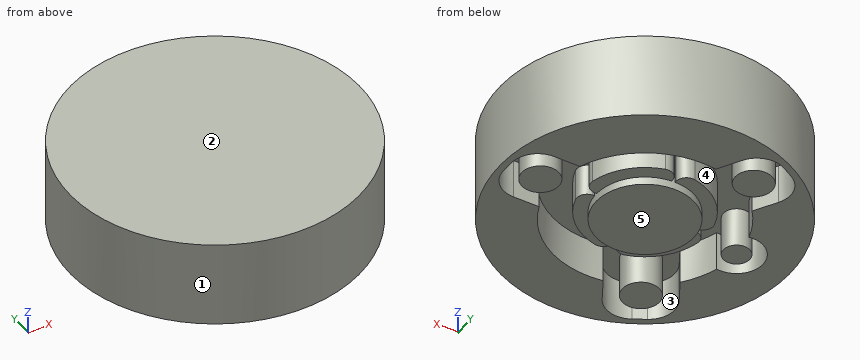
```python
from build123d import *

# Parameters (mm, degrees)
CYLINDER040_R     = 1
CYLINDER040_DEPTH = 10
CYLINDER037_R     = 3.7
CYLINDER037_DEPTH = 10
CYLINDER038_W     = 4.7
CYLINDER038_H     = 10
CYLINDER038_ANGLE = 86
FILLET003_R       = 0.79
ARRAY006_COUNT    = 4
CYLINDER036_R     = 1.4
CYLINDER036_DEPTH = 10
ARRAY004_COUNT    = 3
BOX003_W          = 10
BOX003_H          = 5
BOX003_DEPTH      = 3
FILLET002_R       = 2
ARRAY005_COUNT    = 3
CYLINDER035_R     = 7
CYLINDER035_DEPTH = 3
CYLINDER039_R     = 2
CYLINDER039_DEPTH = 3
CYLINDER042_R     = 11
CYLINDER042_DEPTH = 6.5


with BuildPart() as cylinder022:
    # Cylinder040 → Cylinder040 (new body)
    with BuildSketch(Plane(origin=(-7, 0, 0), x_dir=(1, 0, 0), z_dir=(0, 0, 1))):
        Circle(CYLINDER040_R)
    extrude(amount=CYLINDER040_DEPTH)


with BuildPart() as mountplateinnerhole002:
    # Cylinder037 → Cylinder037 (new body)
    with BuildSketch(Plane.XY):
        Circle(CYLINDER037_R)
    extrude(amount=CYLINDER037_DEPTH)


with BuildPart() as array006:
    # Cylinder038 → Cylinder038 (revolve)
    with BuildSketch(Plane(origin=(0, 0, 0.6), x_dir=(1, 0, 0), z_dir=(0, -1, 0))):
        with Locations((2.35, 5)):
            Rectangle(CYLINDER038_W, CYLINDER038_H)
    revolve(axis=Axis((0, 0, 0.6), (0, 0, 1)), revolution_arc=CYLINDER038_ANGLE)

    # Fillet003
    fillet003_edges = [array006.edges().sort_by_distance(p)[0] for p in [
        (0.327855, 4.688551, 5.6),
        (4.7, 0, 5.6),
    ]]
    fillet(fillet003_edges, radius=FILLET003_R)

    # Array006: Array006 ×4 about axis
    array006_axis = Axis((0, 0, 0), (0, 0, 1))


with BuildPart() as array006_1:
    add(array006.part)
    for i in range(1, ARRAY006_COUNT):
        add(array006.part.rotate(array006_axis, i * 360 / ARRAY006_COUNT))


with BuildPart() as fusion011:
    # Cylinder036 → Cylinder036 (new body)
    with BuildSketch(Plane(origin=(8, 0, 0), x_dir=(1, 0, 0), z_dir=(0, 0, 1))):
        Circle(CYLINDER036_R)
    extrude(amount=CYLINDER036_DEPTH)

    # Array004: Fusion011 ×3 about axis
    array004_axis = Axis((0, 0, 0), (0, 0, 1))


with BuildPart() as fusion011_1:
    add(fusion011.part)
    for i in range(1, ARRAY004_COUNT):
        add(fusion011.part.rotate(array004_axis, i * 360 / ARRAY004_COUNT))

    # Fusion011: union Cylinder022, MountPlateInnerHole002, Array006
    add(cylinder022.part)
    add(mountplateinnerhole002.part)
    add(array006_1.part)


with BuildPart() as array005:
    # Box003 → Box003 (new body)
    with BuildSketch(Plane(origin=(0.5, -2.5, 0), x_dir=(1, 0, 0), z_dir=(0, 0, 1))):
        with Locations((5, 2.5)):
            Rectangle(BOX003_W, BOX003_H)
    extrude(amount=BOX003_DEPTH)

    # Fillet002
    fillet002_edges = [array005.edges().sort_by_distance(p)[0] for p in [
        (10.5, -2.5, 1.5),
        (10.5, 2.5, 1.5),
    ]]
    fillet(fillet002_edges, radius=FILLET002_R)

    # Array005: Array005 ×3 about axis
    array005_axis = Axis((0, 0, 0), (0, 0, 1))


with BuildPart() as array005_1:
    add(array005.part)
    for i in range(1, ARRAY005_COUNT):
        add(array005.part.rotate(array005_axis, i * 360 / ARRAY005_COUNT))


with BuildPart() as mountplatebody002:
    # Cylinder035 → Cylinder035 (new body)
    with BuildSketch(Plane.XY):
        Circle(CYLINDER035_R)
    extrude(amount=CYLINDER035_DEPTH)


with BuildPart() as cut011:
    # Cylinder039 → Cylinder039 (new body)
    with BuildSketch(Plane(origin=(-7, 0, 0), x_dir=(1, 0, 0), z_dir=(0, 0, 1))):
        Circle(CYLINDER039_R)
    extrude(amount=CYLINDER039_DEPTH)

    # Fusion010: union Array005, MountPlateBody002
    add(array005_1.part)
    add(mountplatebody002.part)

    # Cut011: cut Fusion011
    add(fusion011_1.part, mode=Mode.SUBTRACT)


with BuildPart() as cut012:
    # Cylinder042 → Cylinder042 (new body)
    with BuildSketch(Plane.XY):
        Circle(CYLINDER042_R)
    extrude(amount=CYLINDER042_DEPTH)

    # Cut012: cut Cut011
    add(cut011.part, mode=Mode.SUBTRACT)


solid = cut012.part
```
Here's how the part is built. I have some questions about the finished solid (model axes, mm). Face numbers are marked on the shaded views. A direction names the side the tool comes from. Coordinates: 2 decimals unless noted, no trailing zeros. Loops run counter-clockwise (first coordinate to the right, second up) from the corner with the lowest first, then second, coordinate; pieces in that order, holes last. Notation, with made-up numbers: (-39.5, 76.25) -> (-2.5, 76.25) arc R17 ccw to (-2.5, 104.25) -> close; hole circle Ø3 at (8.5, 6.5). An arc over 180 degrees is marked (long way). Return JSON: item names as keys, results as strings.
1) I need wall thicknesses on line 1 (Y direction, x = -7, z = 2.1); line 2 (X direction, y = -3.25, z = 1.75); line 3 (X direction, y = 0.5, z = 0.75). Which ranges of each line are inside material? Lowest first, please. Write a range as from..to.
Results below:
{"line 1": "-8.49..-2, -1..1, 2..8.49", "line 2": "-10.51..-6.2, -3.4..3.4, 6.2..10.51", "line 3": "-10.99..-8.94, -7.87..-6.13, -4.33..4.56, 6.69..9.31, 10.5..10.99"}
2) If we section it at D-D, the plane z = 4.5: Write out the boundary of the cut face in (x, y).
Results below:
{"outline": "circle Ø22 at (0, 0)"}
3) For the marked faces 4 and 5, which set-ups out of +Z, -Z, +X, -X, +Y, -Y let a thin tool reach every point of the face, with its end or its side?
Results below:
{"face 4": "-Z", "face 5": "-Z, +X, -X, +Y, -Y"}
4) Will these pins go through, and if not, where does the flat tip stop? pin 1 (1.6 mm diameter, centred on x = 7, z = 2, fed in from -Y); pin 2 (1 mm diameter, centred on y = -2.5, z = 5.5, fed in from +X); pin 3 (0.6 mm diameter, centred on x = 8, z = 1, fed in from +Y).
Results below:
{"pin 1": "y = -9.09", "pin 2": "x = 10.82", "pin 3": "y = 7.86"}
5) Thinking about a two-plate mould opening in X: for the marked faces 1, 2 and 3, which applies, +X half, -X half, draft (parallel to the pull), parting line (faces both ways), or undercut?
Results below:
{"face 1": "parting line", "face 2": "draft", "face 3": "undercut"}
6) If we section it at B-B, the plane x = -7: Write out the boundary of the cut face in (y, z).
Results below:
{"outline": "(-8.49, 0) -> (-2, 0) -> (-2, 3) -> (-1, 3) -> (-1, 0) -> (1, 0) -> (1, 3) -> (2, 3) -> (2, 0) -> (8.49, 0) -> (8.49, 6.5) -> (-8.49, 6.5) -> close"}
7) If we section it at C-C, the plane y = -7.5: Write out the boundary of the cut face in (x, z).
Results below:
{"outline": "(-8.05, 0) -> (-6.64, 0) -> (-6.64, 3) -> (-5.28, 3) -> (-5.28, 0) -> (-2.72, 0) -> (-2.72, 3) -> (-1.44, 3) -> (-1.44, 0) -> (8.05, 0) -> (8.05, 6.5) -> (-8.05, 6.5) -> close"}
8) If we section it at A-A, the plane z = 1: Count the separate pieces of the cut face and the enclosed holes in it, then the cut area to 3 significant figures.
Results below:
{"separate pieces": "6", "enclosed holes": "1", "area": "258 mm²"}
